```python
from build123d import *

# Parameters (mm, degrees)
F0_W     = 50
F0_H     = 50
F0_W_2   = 35
F0_H_2   = 35
F0_R     = 10.55
F1_DEPTH = 5
F2_W     = 35
F2_H     = 35
F2_R     = 10.55
F3_DEPTH = 2
F4_DEPTH = 3.5


with BuildPart() as f1:
    # F0 (on Top) → F1 (new body)
    with BuildSketch(Plane.XY):
        Rectangle(F0_W, F0_H)
        Rectangle(F0_W_2, F0_H_2, mode=Mode.SUBTRACT)
        Rectangle(F0_W_2, F0_H_2)
        Circle(F0_R, mode=Mode.SUBTRACT)
        Circle(F0_R)
    extrude(amount=F1_DEPTH)

    # F2 (on face) → F3 (cut)
    with BuildSketch(Plane.XY.offset(5)):
        Rectangle(F2_W, F2_H)
        Circle(F2_R, mode=Mode.SUBTRACT)
        Circle(F2_R)
    extrude(amount=-F3_DEPTH, mode=Mode.SUBTRACT)

    # F2 (on face) → F4 (cut)
    with BuildSketch(Plane.XY.offset(5)):
        Circle(F2_R)
    extrude(amount=-F4_DEPTH, mode=Mode.SUBTRACT)


solid = f1.part
```
The listing builds one solid part. Answer for the finished solid, in the listing's coordinates (mm). A direction names the side the tool comes from. Give positions to 0.01 mm unless a question says otherwise; leave off trailing zeros. Order: outer loops, then holes, each group sorted by start corner. A loop starts at its lowest first (then second) coordinate and runs counter-clockwise, first axis right, second up.
1) Given P1, Ø2, axis at x = 16, y = 17.5, coming from the -Z side; P2, Ø23, axis at x = -5, y = 4, coming from the +Z side; P3, Ø4, axis at x = -4, y = -6.5, coming from the +Z side, each flat-ended and moving along its own axis, determine where each tip first touches the part or whether it passes through.
Reported:
P1: stops at z = 0
P2: stops at z = 3
P3: stops at z = 1.5
2) Consider line 1 along Y through (x, z) = (0, 2); line 2 along X through (y, z) = (7, 4.55). Determine where each line is inside the solid, lowest interval first.
Reported:
line 1: y = -25 to -10.55, 10.55 to 25
line 2: x = -25 to -17.5, 17.5 to 25
3) For faces 1 (the face through (0, 0, 1.5)), 2 (the face through (0, 0, 0)), determine the directions among +Z, -Z, +X, -X, +Y, -Y from which every point of the face is accessible in a straight line to the end or side of a thin tool.
Reported:
face 1: +Z
face 2: -Z, +X, -X, +Y, -Y
4) Find section C-C on x = 0. Write down the section's boundary in (y, z).
Reported:
outline: (-25, 0) - (25, 0) - (25, 5) - (17.5, 5) - (17.5, 3) - (10.55, 3) - (10.55, 1.5) - (-10.55, 1.5) - (-10.55, 3) - (-17.5, 3) - (-17.5, 5) - (-25, 5) - close
5) Find section A-A on z = 4.05. Write down the section's boundary in (x, y).
Reported:
outline: (-25, -25) - (25, -25) - (25, 25) - (-25, 25) - close; hole (-17.5, -17.5) - (17.5, -17.5) - (17.5, 17.5) - (-17.5, 17.5) - close
6) Determine the mould class of faces 3 (the face through (8, 8, 3)), 4 (the face through (25, 0, 2)), 5 (the face through (0, 17.5, 4)), 6 (the face through (0, 25, 2)) for opening direction Y: pulls with the +Y half, pulls with the -Y half, needs draft (parallel to the pull), parting line crosses it, or undercut.
Reported:
face 3: undercut
face 4: needs draft
face 5: undercut
face 6: pulls with the +Y half
7) Find section B-B on y = 12. Write down the section's boundary in (x, z), then the cut area to 3 significant figures.
Reported:
outline: (-25, 0) - (25, 0) - (25, 5) - (17.5, 5) - (17.5, 3) - (-17.5, 3) - (-17.5, 5) - (-25, 5) - close
area: 180 mm2
